Read the model definition and answer for the solid it produces. Units are mm, in the model's axes. A direction names the side the tool comes from. Give positions to 0.01 mm unless a question says otherwise; leave off trailing zeros. Loops run counter-clockwise (first coordinate to the right, second up) from the corner with the lowest first, then second, coordinate; pieces in that order, holes last.
(1) Find section B-B, the plane x = 70. Write down the section's boundary in (y, z).
(2) Find section C-C, the plane z = 8. Write down the section's boundary in (x, y).
(3) Straight lines are drawn through the part: probe 1 along Z at (x, y) = (88, 15.5); probe 2 along Y at (x, z) = (73, 8.25); probe 3 along Y at (x, z) = (66.5, 7.75). For each, find the intervals that lie inside material, in ascending order.
(4) Which of the six approach directions +Z, -Z, +X, -X, +Y, -Y give full straight-line access (tool end or side, diameter ignored) to faces 1 (the face through (99.987, -1.623, 0.986)), 2 (the face through (73.695, -1.532, 6.437))?
(5) Find section A-A, the plane y = 0. Write down the section's boundary in (x, z).
(6) Each of these flat-tipped pins is pushed along its axis until it touches: P1, Ø1.5, axis at y = 2.5, z = 4, coming from the -X side; P2, Ø1.5, axis at y = -27.5, z = 1.5, coming from the +X side; P3, Ø8, axis at x = 53, y = 1, coming from the +Z side. Where does it stop, or does it pass through?
(7) Find section D-D, the plane x = 53.5. Write down the section's boundary in (y, z), then the cut area to 3 significant figures.
```python
from build123d import *

# Parameters (mm, degrees)
F1_DEPTH = 2
F2_R     = 4
F3_DEPTH = 10
F4_SIZE  = 1


with BuildPart() as f1:
    # F0 (on Top) → F1 (new body)
    with BuildSketch(Plane.XY):
        with BuildLine():
            Line((40, 91.651514), (40, -91.651514))
            ThreePointArc((40, -91.651514), (100, 0), (40, 91.651514))
        make_face()
    extrude(amount=F1_DEPTH)

    # F2 (on face) → F3 (join)
    with BuildSketch(Plane.XY.offset(2)):
        with Locations((70, 0)):
            Circle(F2_R)
    extrude(amount=F3_DEPTH)

    # F4
    f4_edges = [f1.edges().sort_by_distance(p)[0] for p in [
        (66, 0, 12),
    ]]
    chamfer(f4_edges, length=F4_SIZE)


solid = f1.part
```
Entries:
1. outline: (-71.41, 0) - (71.41, 0) - (71.41, 2) - (4, 2) - (4, 11) - (3, 12) - (-3, 12) - (-4, 11) - (-4, 2) - (-71.41, 2) - close
2. outline: circle Ø8 at (70, 0)
3. probe 1: z = 0 to 2
3. probe 2: y = -2.65 to 2.65
3. probe 3: y = -1.94 to 1.94
4. face 1: +Z, -Z, +X
4. face 2: +Z
5. outline: (40, 0) - (100, 0) - (100, 2) - (74, 2) - (74, 11) - (73, 12) - (67, 12) - (66, 11) - (66, 2) - (40, 2) - close
6. P1: stops at x = 66.4
6. P2: stops at x = 96.36
6. P3: stops at z = 2
7. outline: (-84.49, 0) - (84.49, 0) - (84.49, 2) - (-84.49, 2) - close
7. area: 338 mm2
